from build123d import *

# Parameters (mm, degrees)
SKETCH1_R           = 30
SKETCH1_R_2         = 12
SKETCH1_R_3         = 20
BOSS_EXTRUDE1_DEPTH = 100


with BuildPart() as part:
    # Sketch1 → Boss-Extrude1 (new body)
    with BuildSketch(Plane(origin=(0, 0, 0), x_dir=(1, 0, 0), z_dir=(0, 1, 0))):
        with BuildLine():
            Line((-84.293098865, -116), (83.706901135, -116))
            Line((83.706901135, -116), (83.706901135, -92))
            Line((83.706901135, -92), (55.706901135, -92))
            ThreePointArc((55.706901135, -92), (51.464260447, -90.242640687), (49.706901135, -86))
            Line((49.706901135, -86), (49.706901135, -38.271491466))
            ThreePointArc((49.706901135, -38.271491466), (50.585759142, -35.440204006), (52.913376606, -33.604236409))
            ThreePointArc((52.913376606, -33.604236409), (69.672222345, -20.385269709), (76, 0))
            ThreePointArc((76, 0), (70.285133563, 28.91366459), (54, 53.478967828))
            ThreePointArc((54, 53.478967828), (39.883656587, 86.745545299), (39.361130578, 122.87950847))
            ThreePointArc((39.361130578, 122.87950847), (0, 170), (-39.361130578, 122.87950847))
            ThreePointArc((-39.361130578, 122.87950847), (-39.883656587, 86.745545299), (-54, 53.478967828))
            ThreePointArc((-54, 53.478967828), (-70.285133563, 28.91366459), (-76, 0))
            ThreePointArc((-76, 0), (-69.827932589, -20.156746698), (-53.428086809, -33.401893429))
            ThreePointArc((-53.428086809, -33.401893429), (-51.15033045, -35.241497142), (-50.293098865, -38.041045294))
            Line((-50.293098865, -38.041045294), (-50.293098865, -86))
            ThreePointArc((-50.293098865, -86), (-52.050458178, -90.242640687), (-56.293098865, -92))
            Line((-56.293098865, -92), (-84.293098865, -92))
            Line((-84.293098865, -92), (-84.293098865, -116))
        make_face()
        with Locations(Location((0.719405778, -64, 0), (0, 0, 270))):
            Circle(SKETCH1_R, mode=Mode.SUBTRACT)
        with Locations(Location((0, 0, 0), (0, 0, 270))):
            Circle(SKETCH1_R_2, mode=Mode.SUBTRACT)
        with Locations(Location((0, 130, 0), (0, 0, 270))):
            Circle(SKETCH1_R_3, mode=Mode.SUBTRACT)
        with BuildLine():
            ThreePointArc((-54, 0), (-40, -14), (-26, 0))
            ThreePointArc((-26, 0), (0, 26), (26, 0))
            ThreePointArc((26, 0), (40, -14), (54, 0))
            ThreePointArc((54, 0), (0, 54), (-54, 0))
        make_face(mode=Mode.SUBTRACT)
    extrude(amount=BOSS_EXTRUDE1_DEPTH)


solid = part.part
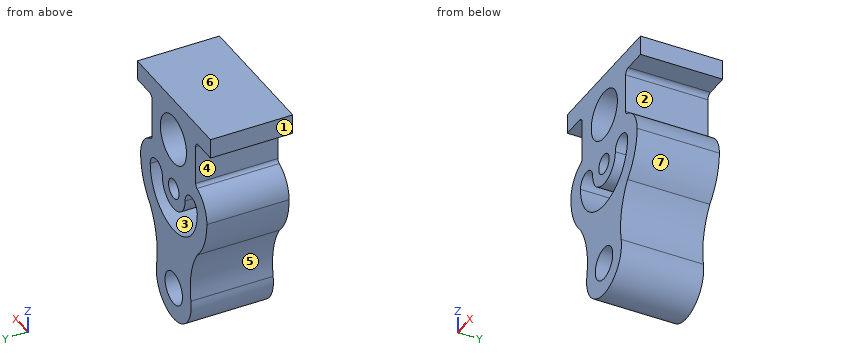
Could you check a few things on this model? Use its own coordinates, in mm. Face numbers are marked on the shaded views. A direction names the side the tool comes from. Coordinates: 2 decimals unless noted, no trailing zeros. Write each loop counter-clockwise with the first axis right and the second up, starting at its lowest first coordinate (ties: lowest second). Pieces come first, ordered by that corner, then holes. Notation, with made-up numbers: M 33,10 L 88,10 A37 cw 88,47 Z; hole C 12,30.25 d11. An arc over 180 degrees is marked long. One line per question, with ' | ' between items.
1) Imagine slicing it at A-A, the plane z = -130. Write out the boundary of the cut face in (x, y), and give its area (3 significant figures).
Checks:
outline: M -40,0 L -20,0 L -20,100 L -40,100 Z; M 20,0 L 40,0 L 40,100 L 20,100 Z | area: 4,000 mm²
2) If we mould it in two halves opening along Z, with no side actions, what happens to the marked faces 5, 6 and 7? For each: released by +Z, released by -Z, zero draft, split by the parting line, or undercut.
Checks:
face 5: undercut | face 6: released by +Z | face 7: released by -Z
3) Imagine slicing it at C-C, the plane y = 66.5. Write out the boundary of the cut face in (x, z).
Checks:
outline: M -84.29,92 L -56.29,92 A6 cw -50.29,86 L -50.29,38.04 A5 cw -53.43,33.4 A36 ccw -76,0 A76 ccw -54,-53.48 A94 cw -39.36,-122.88 A40 ccw long 39.36,-122.88 A94 cw 54,-53.48 A76 ccw 76,0 A36 ccw 52.91,33.6 A5 cw 49.71,38.27 L 49.71,86 A6 cw 55.71,92 L 83.71,92 L 83.71,116 L -84.29,116 Z; hole M -54,0 A54 ccw 54,0 A14 ccw 26,0 A26 cw -26,0 A14 ccw Z; hole C 0.72,64 d60; hole C 0,-130 d40; hole C 0,0 d24
4) Imagine slicing it at D-D, the plane z = 4.5. Write out the boundary of the cut face in (x, y).
Checks:
outline: M -75.72,0 L -53.26,0 L -53.26,100 L -75.72,100 Z; M -26.74,0 L -11.12,0 L -11.12,100 L -26.74,100 Z; M 11.12,0 L 26.74,0 L 26.74,100 L 11.12,100 Z; M 53.26,0 L 75.72,0 L 75.72,100 L 53.26,100 Z
5) I need wall thicknesses on probe 1 along X at (y, z) = (47, 64); probe 2 along X at (y, z) = (64, -130); probe 3 along Z at (x, y) = (28, 40). Which ranges of each line are inside material? Lowest first, please. Write a range as [from, to].
Checks:
probe 1: [-50.29, -29.28], [30.72, 49.71] | probe 2: [-40, -20], [20, 40] | probe 3: [-158.57, -46.17], [7.21, 51.52], [76.48, 116]
6) For the marked faces 1, 2, 3 and 4, which set-ups out of +Z, -Z, +X, -X, +Y, -Y let a thin tool reach every point of the face, with its end or its side?
Checks:
face 1: +Z, -Z, -X, +Y, -Y | face 2: +X, +Y, -Y | face 3: +Y, -Y | face 4: -X, +Y, -Y
7) For pin 1 Ø22.5 at (x, y) = (-67, 56.5) entering from -Z; pin 2 Ø1.5 at (y, z) = (41.5, -49) entering from +X; pin 3 Ø14 at (x, y) = (69.5, 29) entering from -Z, each with a flat end and sliding along its axis, tell me the tip position at first contact or that it passes through.
Checks:
pin 1: z = -51.65 | pin 2: x = 58.72 | pin 3: z = -43.24
8) Imagine slicing it at B-B, the plane x = 72.5. Write out the boundary of the cut face in (y, z), and give its area (3 significant figures).
Checks:
outline: M 0,-22.8 L 100,-22.8 L 100,15.48 L 0,15.48 Z; M 0,92 L 100,92 L 100,116 L 0,116 Z | area: 6,230 mm²
